```python
from build123d import *

# Parameters (mm, degrees)
SKETCH1_W           = 69
SKETCH1_H           = 20
BOSS_EXTRUDE1_DEPTH = 0.7
BOSS_EXTRUDE2_DEPTH = 0.25


with BuildPart() as part:
    # Sketch1 → Boss-Extrude1 (new body)
    with BuildSketch(Plane(origin=(0, 0, 0), x_dir=(1, 0, 0), z_dir=(0, 1, 0))):
        Rectangle(SKETCH1_W, SKETCH1_H)
    extrude(amount=BOSS_EXTRUDE1_DEPTH)

    # Sketch2 → Boss-Extrude2 (add)
    with BuildSketch(Plane(origin=(0, 0.7, 0), x_dir=(1, 0, 0), z_dir=(0, 1, 0))):
        with BuildLine():
            Line((-26.9, -5.5), (-16.9, -5.5))
            ThreePointArc((-16.9, -5.5), (-16.546446609, -5.353553391), (-16.4, -5))
            Line((-16.4, -5), (-16.4, 5))
            ThreePointArc((-16.4, 5), (-16.546446609, 5.353553391), (-16.9, 5.5))
            Line((-16.9, 5.5), (-26.9, 5.5))
            ThreePointArc((-26.9, 5.5), (-27.253553391, 5.353553391), (-27.4, 5))
            Line((-27.4, 5), (-27.4, -5))
            ThreePointArc((-27.4, -5), (-27.253553391, -5.353553391), (-26.9, -5.5))
        make_face()
        with BuildLine():
            Line((-12.3, -5.5), (-2.3, -5.5))
            ThreePointArc((-2.3, -5.5), (-1.946446609, -5.353553391), (-1.8, -5))
            Line((-1.8, -5), (-1.8, 5))
            ThreePointArc((-1.8, 5), (-1.946446609, 5.353553391), (-2.3, 5.5))
            Line((-2.3, 5.5), (-12.3, 5.5))
            ThreePointArc((-12.3, 5.5), (-12.653553391, 5.353553391), (-12.8, 5))
            Line((-12.8, 5), (-12.8, -5))
            ThreePointArc((-12.8, -5), (-12.653553391, -5.353553391), (-12.3, -5.5))
        make_face()
        with BuildLine():
            Line((2.3, -5.5), (12.3, -5.5))
            ThreePointArc((12.3, -5.5), (12.653553391, -5.353553391), (12.8, -5))
            Line((12.8, -5), (12.8, 5))
            ThreePointArc((12.8, 5), (12.653553391, 5.353553391), (12.3, 5.5))
            Line((12.3, 5.5), (2.3, 5.5))
            ThreePointArc((2.3, 5.5), (1.946446609, 5.353553391), (1.8, 5))
            Line((1.8, 5), (1.8, -5))
            ThreePointArc((1.8, -5), (1.946446609, -5.353553391), (2.3, -5.5))
        make_face()
        with BuildLine():
            Line((16.9, -5.5), (26.9, -5.5))
            ThreePointArc((26.9, -5.5), (27.253553391, -5.353553391), (27.4, -5))
            Line((27.4, -5), (27.4, 5))
            ThreePointArc((27.4, 5), (27.253553391, 5.353553391), (26.9, 5.5))
            Line((26.9, 5.5), (16.9, 5.5))
            ThreePointArc((16.9, 5.5), (16.546446609, 5.353553391), (16.4, 5))
            Line((16.4, 5), (16.4, -5))
            ThreePointArc((16.4, -5), (16.546446609, -5.353553391), (16.9, -5.5))
        make_face()
    extrude(amount=BOSS_EXTRUDE2_DEPTH)


solid = part.part
```
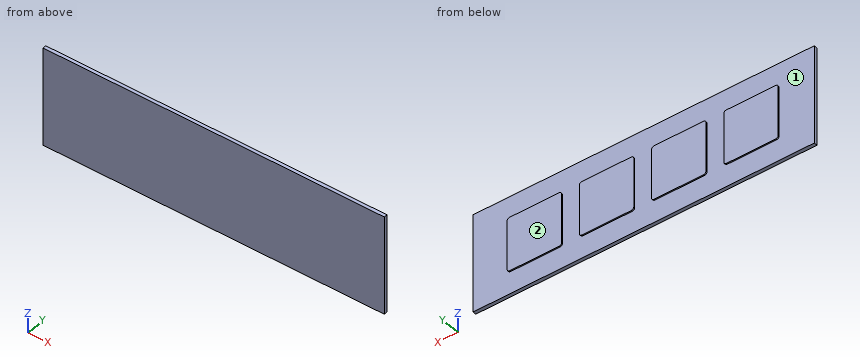
Design review of the part built by this model. Coordinates are the model's own, in mm. Face numbers are marked on the shaded views. Coordinates: 2 decimals unless noted, no trailing zeros. Order: outer loops, then holes, each group sorted by start corner. A loop starts at its lowest first (then second) coordinate and runs counter-clockwise, first axis right, second up. Notation, with made-up numbers: (74.25, 43.5) - (99.25, 43.5) arc R36 cw to (99.25, 77.5) - close; hole circle Ø3 at (5.5, -16). An arc over 180 degrees is marked (long way). One line per question, with ' | ' between items.
Q1. Consider section A-A, the plane x = -22.5. Give the boundary of the cut face in (y, z).
Answer key:
outline: (0, -10) - (0.7, -10) - (0.7, -5.5) - (0.95, -5.5) - (0.95, 5.5) - (0.7, 5.5) - (0.7, 10) - (0, 10) - close
Q2. Consider section B-B, the plane z = 0.25. Give the boundary of the cut face in (x, y), then the cut area to 3 significant figures.
Answer key:
outline: (-34.5, 0) - (34.5, 0) - (34.5, 0.7) - (27.4, 0.7) - (27.4, 0.95) - (16.4, 0.95) - (16.4, 0.7) - (12.8, 0.7) - (12.8, 0.95) - (1.8, 0.95) - (1.8, 0.7) - (-1.8, 0.7) - (-1.8, 0.95) - (-12.8, 0.95) - (-12.8, 0.7) - (-16.4, 0.7) - (-16.4, 0.95) - (-27.4, 0.95) - (-27.4, 0.7) - (-34.5, 0.7) - close | area: 59.3 mm2
Q3. Consider section C-C, the plane z = -7. Give the boundary of the cut face in (x, y).
Answer key:
outline: (-34.5, 0) - (34.5, 0) - (34.5, 0.7) - (-34.5, 0.7) - close
Q4. The part is to be moulded in two halves that separate along X. For the marked faces 1 and 2, say which applies: +X half, -X half, draft (parallel to the pull), parting line (faces both ways), or undercut.
Answer key:
face 1: undercut | face 2: draft
Q5. To check wall thickness, follow line 1 along X through (y, z) = (0.8, -3.75); line 2 along Y through (x, z) = (22.5, 7); line 3 along Z through (x, y) = (-3.5, 0.75). State the ranges of each line that lie inside material, in increasing order.
Answer key:
line 1: x = -27.4 to -16.4, -12.8 to -1.8, 1.8 to 12.8, 16.4 to 27.4 | line 2: y = 0 to 0.7 | line 3: z = -5.5 to 5.5
